Work out the finished part from the listing and answer in its coordinate system (mm). Coordinates: 2 decimals unless noted, no trailing zeros. Loops run counter-clockwise (first coordinate to the right, second up) from the corner with the lowest first, then second, coordinate; pieces in that order, holes last. Notation, with made-up numbers: (1, 27) - (6, 27) arc R24 cw to (6, 48) - close; hole circle Ø9 at (-33, 1). An arc over 180 degrees is marked (long way). Write each question's results on one line, items separated by ' | '. Start each with the question number.
Item 1: Section C-C, the plane x = -148.5 is taken. Write down the section's boundary in (y, z).
Item 2: Section D-D, the plane y = -5 is taken. Write down the section's boundary in (x, z).
Item 3: Each of these flat-tipped pins is pushed along its axis until it touches: pin 1 Ø6 at (y, z) = (-6.5, -10.5) entering from -X; pin 2 Ø3 at (x, z) = (-158, -47) entering from -Y; pin 3 Ø12 at (x, z) = (66, -76) entering from -Y. Where does it stop, or does it pass through?
Item 4: Section B-B, the plane y = 13.5 is taken. Write down the section's boundary in (x, z), plus the area to 3 significant figures.
Item 5: Consider probe 1 along Y at (x, z) = (137, 14); probe 2 along X at (y, z) = (-25, -8.5); probe 3 along X at (y, z) = (28.5, 25.5). Determine where each line is inside the solid, lowest interval first. Write a range as [from, to].
Item 6: For a pull along X with two mould halves and no side action, classify faces 1 (the face through (15, -67.515, -10)), 2 (the face through (-19.524, -51.047, -17.565)), 3 (the face through (0.66, -50.58, -28.215)) as +X half, -X half, draft (parallel to the pull), parting line (faces both ways), or undercut.
Item 7: Section A-A, the plane x = 0 is taken. Write down the section's boundary in (y, z), plus the area to 3 significant figures.
from build123d import *

# Parameters (mm, degrees)
ESQUISSE4_W             = 400
ESQUISSE4_H             = 131.578163935
ESQUISSE4_H_2           = 129.819251152
ENL_V_MAT_EXTRU_1_DEPTH = 10
BOSS_EXTRU_2_DEPTH      = 5


with BuildPart() as part:
    # Esquisse1 → Révolution3 (revolve)
    with BuildSketch(Plane(origin=(0, 0, 0), x_dir=(0, 0, -1), z_dir=(1, 0, 0))):
        with BuildLine():
            Line((-1.770428016, -67.515182568), (-1.770428016, -34.11154345))
            ThreePointArc((-1.770428016, -34.11154345), (-31.059749897, 36.599134669), (-101.770428016, 65.88845655))
            Line((-101.770428016, 65.88845655), (-186.770428016, 65.88845655))
            Line((-186.770428016, 65.88845655), (-186.770428016, 60.88845655))
            Line((-186.770428016, 60.88845655), (-101.770428016, 60.88845655))
            ThreePointArc((-101.770428016, 60.88845655), (-34.595283803, 33.063600763), (-6.770428016, -34.11154345))
            Line((-6.770428016, -34.11154345), (-6.770428016, -67.515182568))
            Line((-6.770428016, -67.515182568), (-1.770428016, -67.515182568))
        make_face()
    revolve(axis=Axis((0, -67.515182568, -13.229571984), (0, 1, 0)))

    # Esquisse4 → Enlèv. mat.-Extru.1 (cut)
    with BuildSketch(Plane(origin=(0, 65.88845655, 0), x_dir=(1, 0, 0), z_dir=(0, 1, 0))):
        with Locations((0, -142.559509983)):
            Rectangle(ESQUISSE4_W, ESQUISSE4_H)
        with Locations((0, 168.13919756)):
            Rectangle(ESQUISSE4_W, ESQUISSE4_H_2)
    extrude(amount=-ENL_V_MAT_EXTRU_1_DEPTH, mode=Mode.SUBTRACT)

    # Esquisse5 → Boss.-Extru.2 (add)
    with BuildSketch(Plane(origin=(0, 65.88845655, 0), x_dir=(1, 0, 0), z_dir=(0, 1, 0))):
        Polygon((-200, 13.229571984), (-200, 103.229571984), (-178.605710995, 103.229571984), (-178.605710995, -76.770428016), (-200, -76.770428016), align=None)
        Polygon((200, 13.229571984), (200, 103.229571984), (178.605710995, 103.229571984), (178.605710995, -76.770428016), (200, -76.770428016), align=None)
    extrude(amount=-BOSS_EXTRU_2_DEPTH)


solid = part.part
Answer key:
1) outline: (60.89, -103.23) - (65.89, -103.23) - (65.89, 76.77) - (60.89, 76.77) - close
2) outline: circle Ø49.14 at (0, -13.23); hole circle Ø38.66 at (0, -13.23)
3) pin 1: stops at x = -24.96 | pin 2: stops at y = 60.89 | pin 3: stops at y = 56.05
4) outline: circle Ø65.58 at (0, -13.23); hole circle Ø54.12 at (0, -13.23) | area: 1,080 mm^2
5) probe 1: y = [60.89, 65.89] | probe 2: x = [-19.88, -14.67], [14.67, 19.88] | probe 3: x = [-19.92, 19.92]
6) face 1: draft | face 2: parting line | face 3: undercut
7) outline: (-67.52, -33.23) - (-34.11, -33.23) arc R95 cw to (57.54, -103.23) - (62.71, -103.23) arc R100 ccw to (-34.11, -28.23) - (-67.52, -28.23) - close; (-67.52, 1.77) - (-34.11, 1.77) arc R100 ccw to (62.71, 76.77) - (57.54, 76.77) arc R95 cw to (-34.11, 6.77) - (-67.52, 6.77) - close | area: 1,610 mm^2
